Check sheet for the modelled part. Datum: model origin and axes. Units: mm. Face numbers are marked on the shaded views. A direction names the side the tool comes from. Coordinates: 2 decimals unless noted, no trailing zeros. Write each loop counter-clockwise with the first axis right and the second up, starting at its lowest first coordinate (ties: lowest second). Pieces come first, ordered by that corner, then holes. Notation, with made-up numbers: (71.25, 59.25) - (90.25, 59.25) arc R19 cw to (90.25, 85.25) - close; hole circle Ø10 at (81, 48). An arc over 180 degrees is marked (long way). Write each question's results on one line, items separated by ' | '.
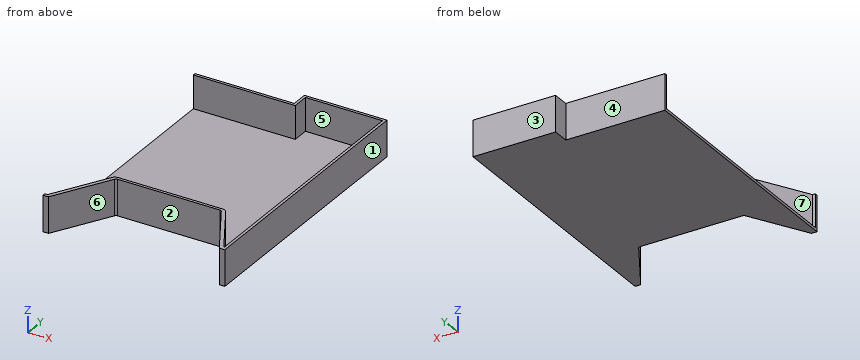
from build123d import *

# Parameters (mm, degrees)
F1_DEPTH = 165.1
F2_DEPTH = 12.7
F0_W     = 12.7
F0_H     = 1117.6
F3_DEPTH = 12.7


with BuildPart() as f1:
    # F0 (on Top) → F1 (new body)
    with BuildSketch(Plane.XY):
        with BuildLine():
            Line((342.9, -361.927737), (368.3, -361.927737))
            Line((368.3, -361.927737), (368.3, 857.272263))
            Line((368.3, 857.272263), (-12.7, 857.272263))
            Line((-12.7, 857.272263), (-12.7, 781.072263))
            Line((-12.7, 781.072263), (-469.9, 781.072263))
            Line((-469.9, 781.072263), (-469.9, 768.372263))
            Line((-469.9, 768.372263), (-457.2, 768.372263))
            Line((-457.2, 768.372263), (0, 768.372263))
            Line((0, 768.372263), (0, 819.172263))
            Line((0, 819.172263), (0, 844.572263))
            Line((0, 844.572263), (355.6, 844.572263))
            Line((355.6, 844.572263), (355.6, -349.227737))
            Line((355.6, -349.227737), (211.822605, -100.197983))
            ThreePointArc((211.822605, -100.197983), (202.52556, -90.900938), (189.82556, -87.497983))
            Line((189.82556, -87.497983), (-291.42556, -87.497983))
            ThreePointArc((-291.42556, -87.497983), (-304.12556, -90.900938), (-313.422605, -100.197983))
            Line((-313.422605, -100.197983), (-457.2, -349.227737))
            Line((-457.2, -349.227737), (-469.9, -349.227737))
            Line((-469.9, -349.227737), (-469.9, -361.927737))
            Line((-469.9, -361.927737), (-444.5, -361.927737))
            Line((-444.5, -361.927737), (-297.056431, -106.547983))
            ThreePointArc((-297.056431, -106.547983), (-292.407908, -101.899461), (-286.057908, -100.197983))
            Line((-286.057908, -100.197983), (184.457908, -100.197983))
            ThreePointArc((184.457908, -100.197983), (190.807908, -101.899461), (195.456431, -106.547983))
            Line((195.456431, -106.547983), (342.9, -361.927737))
        make_face()
    extrude(amount=F1_DEPTH)

    # F0 (on Top) → F2 (join)
    with BuildSketch(Plane.XY):
        with BuildLine():
            Line((0, 768.372263), (-457.2, 768.372263))
            Line((-457.2, 768.372263), (-457.2, -349.227737))
            Line((-457.2, -349.227737), (-313.422605, -100.197983))
            ThreePointArc((-313.422605, -100.197983), (-304.12556, -90.900938), (-291.42556, -87.497983))
            Line((-291.42556, -87.497983), (189.82556, -87.497983))
            ThreePointArc((189.82556, -87.497983), (202.52556, -90.900938), (211.822605, -100.197983))
            Line((211.822605, -100.197983), (355.6, -349.227737))
            Line((355.6, -349.227737), (355.6, 844.572263))
            Line((355.6, 844.572263), (0, 844.572263))
            Line((0, 844.572263), (0, 819.172263))
            Line((0, 819.172263), (0, 768.372263))
        make_face()
    extrude(amount=F2_DEPTH)

    # F0 (on Top) → F3 (join)
    with BuildSketch(Plane.XY):
        with Locations((-463.55, 209.572263)):
            Rectangle(F0_W, F0_H)
    extrude(amount=F3_DEPTH)


solid = f1.part
1. Sectioned sample at A-A (y = -149). Record the cut outline in (x, z).
Values follow:
outline: (-469.9, 0) - (-321.57, 0) - (-321.57, 165.1) - (-341.6, 165.1) - (-341.6, 12.7) - (-469.9, 12.7) - close; (219.97, 0) - (368.3, 0) - (368.3, 165.1) - (355.6, 165.1) - (355.6, 12.7) - (240, 12.7) - (240, 165.1) - (219.97, 165.1) - close
2. Material ranges on L1, parallel to Y at x = -216.5, z = 141.5; L2, parallel to Y at x = 72.5, z = 15.5; L3, parallel to X at y = -57, z = 89, recorded low to high. Write a range as [from, to].
Values follow:
L1: y = [-100.2, -87.5], [768.37, 781.07] | L2: y = [-100.2, -87.5], [844.57, 857.27] | L3: x = [355.6, 368.3]
3. Access from +Z, -Z, +X, -X, +Y, -Y to the whole of each face (thin tool, end or side, straight path). Record for the marked faces 4, 5, 6 and 7.
Values follow:
face 4: +Z, -Z, -X, +Y | face 5: +Z | face 6: +Z, -Z, -Y | face 7: +Z, -X
4. Sectioned sample at D-D (y = 137). Record the cut outline in (x, z).
Values follow:
outline: (-469.9, 0) - (368.3, 0) - (368.3, 165.1) - (355.6, 165.1) - (355.6, 12.7) - (-469.9, 12.7) - close
5. Sectioned sample at B-B (x = 95.5). Record the cut outline in (y, z), then the cut area to 3 significant figures.
Values follow:
outline: (-100.2, 0) - (857.27, 0) - (857.27, 165.1) - (844.57, 165.1) - (844.57, 12.7) - (-87.5, 12.7) - (-87.5, 165.1) - (-100.2, 165.1) - close | area: 16,000 mm^2
6. Draft check along X on the marked faces 1, 2 and 3. Enter one of: pulls with the +X half, pulls with the -X half, needs draft (parallel to the pull), parting line crosses it, or undercut.
Values follow:
face 1: pulls with the +X half | face 2: undercut | face 3: needs draft
7. Sectioned sample at C-C (z = 79.5). Record the cut outline in (x, y).
Values follow:
outline: (-469.9, -361.93) - (-444.5, -361.93) - (-297.06, -106.55) arc R12.7 cw to (-286.06, -100.2) - (184.46, -100.2) arc R12.7 cw to (195.46, -106.55) - (342.9, -361.93) - (368.3, -361.93) - (368.3, 857.27) - (-12.7, 857.27) - (-12.7, 781.07) - (-469.9, 781.07) - (-469.9, 768.37) - (0, 768.37) - (0, 844.57) - (355.6, 844.57) - (355.6, -349.23) - (211.82, -100.2) arc R25.4 ccw to (189.83, -87.5) - (-291.43, -87.5) arc R25.4 ccw to (-313.42, -100.2) - (-457.2, -349.23) - (-469.9, -349.23) - close
8. Go/stop test with flat-tipped pins: pin 1 (12 mm diameter, centred on x = -141.5, y = 122.5, fed in from +Z); pin 2 (23 mm diameter, centred on y = 810.5, z = 50, fed in from -X); pin 3 (4 mm diameter, centred on x = -266, z = 56.5, fed in from -Y). Record where each tip stops, or that it passes through.
Values follow:
pin 1: stops at z = 12.7 | pin 2: stops at x = -12.7 | pin 3: stops at y = -100.2
